```python
from build123d import *

# Parameters (mm, degrees)
F0_W     = 6.9
F0_H     = 8
F1_DEPTH = 3
F2_W     = 2.8
F2_H     = 0.5
F2_W_2   = 0.5
F2_H_2   = 1.7
F3_DEPTH = 1


with BuildPart() as f1:
    # F0 (on Front) → F1 (new body)
    with BuildSketch(Plane.XZ):
        with Locations((3.45, -4)):
            Rectangle(F0_W, F0_H)
    extrude(amount=F1_DEPTH)

    # F2 (on face) → F3 (cut)
    with BuildSketch(Plane.XZ.offset(3)):
        with Locations((3.45, -2.15)):
            Rectangle(F2_W, F2_H)
        with Locations((3.45, -5.85)):
            Rectangle(F2_W, F2_H)
        with Locations((3.45, -4)):
            Rectangle(F2_W, F2_H)
        with Locations((1.6, -5)):
            Rectangle(F2_W_2, F2_H_2)
        with Locations((1.6, -3)):
            Rectangle(F2_W_2, F2_H_2)
        with Locations((5.3, -5)):
            Rectangle(F2_W_2, F2_H_2)
        with Locations((5.3, -3)):
            Rectangle(F2_W_2, F2_H_2)
    extrude(amount=-F3_DEPTH, mode=Mode.SUBTRACT)


solid = f1.part
```
Can you work these out from the model? Positions are in its coordinate system, mm. A direction names the side the tool comes from. Give positions to 0.01 mm unless a question says otherwise; leave off trailing zeros. Loops run counter-clockwise (first coordinate to the right, second up) from the corner with the lowest first, then second, coordinate; pieces in that order, holes last. Notation, with made-up numbers: M 2,-21.5 L 19,-21.5 A20 ccw 19,13.5 Z; hole C 57,76 d11. An arc over 180 degrees is marked long. One line per question, with ' | ' between items. Start each with the question number.
Q1. If we mould it in two halves opening along X, with no side actions, what happens to faces 3 (the flat face through (6.9, -1, -4)), 4 (the flat face through (3, -3, -5)), 5 (the flat face through (3.4, -2.5, -2.4))? For each: +X half, -X half, draft (parallel to the pull), parting line (faces both ways), or undercut.
Q2. If we section it at B-B (y = -2.2): State how many separate pieces and enclosed holes the cut face has, plus the area to 3 significant figures.
Q3. If we section it at C-C (x = 1.5): Please give me the cut outline in (y, z).
Q4. If we section it at D-D (z = -2.25): Please give me the cut outline in (x, y).
Q5. For faces 1 (the flat face through (1.35, -2.5, -5)), 2 (the flat face through (3, -1, -8)), which set-ups out of +Z, -Z, +X, -X, +Y, -Y let a thin tool reach every point of the face, with its end or its side?
Q6. If we section it at A-A (z = -4.5): Please give me the cut outline in (x, y).
Computed:
1) face 3: +X half | face 4: draft | face 5: undercut
2) separate pieces: 1 | enclosed holes: 7 | area: 47.6 mm²
3) outline: M -3,-8 L 0,-8 L 0,0 L -3,0 L -3,-2.15 L -2,-2.15 L -2,-3.85 L -3,-3.85 L -3,-4.15 L -2,-4.15 L -2,-5.85 L -3,-5.85 Z
4) outline: M 0,-3 L 1.35,-3 L 1.35,-2 L 1.85,-2 L 1.85,-3 L 2.05,-3 L 2.05,-2 L 4.85,-2 L 4.85,-3 L 5.05,-3 L 5.05,-2 L 5.55,-2 L 5.55,-3 L 6.9,-3 L 6.9,0 L 0,0 Z
5) face 1: -Y | face 2: -Z, +X, -X, +Y, -Y
6) outline: M 0,-3 L 1.35,-3 L 1.35,-2 L 1.85,-2 L 1.85,-3 L 5.05,-3 L 5.05,-2 L 5.55,-2 L 5.55,-3 L 6.9,-3 L 6.9,0 L 0,0 Z
